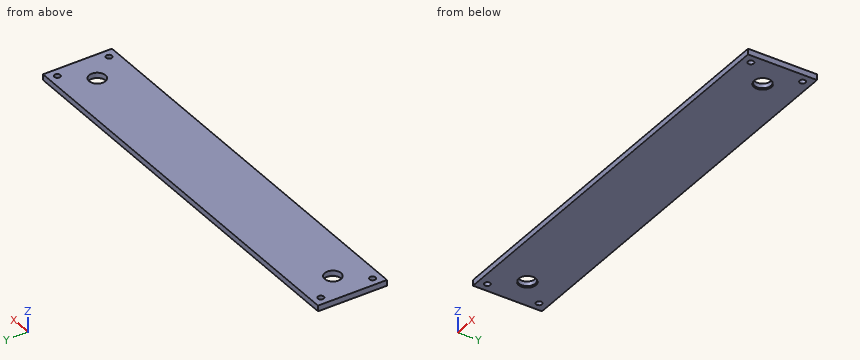
from build123d import *

# Parameters (mm, degrees)
SKETCH1_W           = 360
SKETCH1_H           = 60
SKETCH1_R           = 7.1
BOSS_EXTRUDE1_DEPTH = 4
SKETCH2_W           = 360
SKETCH2_H           = 60
SKETCH2_R           = 7.6
BOSS_EXTRUDE2_DEPTH = 1
CUT_EXTRUDE1_REACH  = 337.423
SKETCH3_R           = 2.55


with BuildPart() as part:
    # Sketch1 → Boss-Extrude1 (new body)
    with BuildSketch(Plane.XY):
        with Locations((-154.041275094, 0)):
            Rectangle(SKETCH1_W, SKETCH1_H)
        Circle(SKETCH1_R, mode=Mode.SUBTRACT)
        with Locations((-308.082550187, -0.2)):
            Circle(SKETCH1_R, mode=Mode.SUBTRACT)
    extrude(amount=-BOSS_EXTRUDE1_DEPTH)

    # Sketch2 → Boss-Extrude2 (add)
    with BuildSketch(Plane(origin=(0, 0, -4), x_dir=(-1, 0, 0), z_dir=(0, 0, -1))):
        with Locations((154.041275094, 0)):
            Rectangle(SKETCH2_W, SKETCH2_H)
        Circle(SKETCH2_R, mode=Mode.SUBTRACT)
        with Locations(Location((308.082550187, 0, 0), (0, 0, 180))):
            Circle(SKETCH2_R, mode=Mode.SUBTRACT)
    extrude(amount=BOSS_EXTRUDE2_DEPTH)

    # Sketch3 → Cut-Extrude1 (cut, up to next)
    with BuildSketch(Plane(origin=(0, 0, -5), x_dir=(-1, 0, 0), z_dir=(0, 0, -1)), mode=Mode.PRIVATE) as cut_extrude1_sk1:
        with Locations((326.53392807, -22.492652976)):
            Circle(SKETCH3_R)
    cut_extrude1_tool1 = extrude(cut_extrude1_sk1.sketch, amount=-CUT_EXTRUDE1_REACH, mode=Mode.PRIVATE) & part.part
    # Sketch3 → Cut-Extrude1 (cut, up to next)
    with BuildSketch(Plane(origin=(0, 0, -5), x_dir=(-1, 0, 0), z_dir=(0, 0, -1)), mode=Mode.PRIVATE) as cut_extrude1_sk2:
        with Locations((326.53392807, 22.492652976)):
            Circle(SKETCH3_R)
    cut_extrude1_tool2 = extrude(cut_extrude1_sk2.sketch, amount=-CUT_EXTRUDE1_REACH, mode=Mode.PRIVATE) & part.part
    # Sketch3 → Cut-Extrude1 (cut, up to next)
    with BuildSketch(Plane(origin=(0, 0, -5), x_dir=(-1, 0, 0), z_dir=(0, 0, -1)), mode=Mode.PRIVATE) as cut_extrude1_sk3:
        with Locations(Location((-18.451377883, -22.492652976, 0), (0, 0, 180))):
            Circle(SKETCH3_R)
    cut_extrude1_tool3 = extrude(cut_extrude1_sk3.sketch, amount=-CUT_EXTRUDE1_REACH, mode=Mode.PRIVATE) & part.part
    # Sketch3 → Cut-Extrude1 (cut, up to next)
    with BuildSketch(Plane(origin=(0, 0, -5), x_dir=(-1, 0, 0), z_dir=(0, 0, -1)), mode=Mode.PRIVATE) as cut_extrude1_sk4:
        with Locations((-18.451377883, 22.492652976)):
            Circle(SKETCH3_R)
    cut_extrude1_tool4 = extrude(cut_extrude1_sk4.sketch, amount=-CUT_EXTRUDE1_REACH, mode=Mode.PRIVATE) & part.part
    add(cut_extrude1_tool1.solids().sort_by_distance((-326.533928, -22.492653, -5))[0], mode=Mode.SUBTRACT)
    add(cut_extrude1_tool2.solids().sort_by_distance((-326.533928, 22.492653, -5))[0], mode=Mode.SUBTRACT)
    add(cut_extrude1_tool3.solids().sort_by_distance((18.451378, -22.492653, -5))[0], mode=Mode.SUBTRACT)
    add(cut_extrude1_tool4.solids().sort_by_distance((18.451378, 22.492653, -5))[0], mode=Mode.SUBTRACT)


solid = part.part
Work out the finished part from the listing and answer in its coordinate system (mm). Round coordinates to 2 decimals unless told otherwise and drop trailing zeros. Write each loop counter-clockwise with the first axis right and the second up, starting at its lowest first coordinate (ties: lowest second). Pieces come first, ordered by that corner, then holes. Notation, with made-up numbers: (56, 80.25) - (101, 80.25) arc R24 ccw to (101, 110.25) - close; hole circle Ø3 at (47, 86.5). An arc over 180 degrees is marked (long way). Answer in a Markdown table with one row per item. Add a question column.
1. A cutting plane is placed at B-B, the plane z = -2.75. Determine the outline of the cut face in (x, y).
2. A cutting plane is placed at A-A, the plane x = 0. Determine the outline of the cut face in (y, z).
3. Find the intervals of material crossed by line 1 along X through (y, z) = (0.5, -3); line 2 along X through (y, z) = (-1, -1.85); line 3 along Y through (x, z) = (0, -4.45), in increasing order. Write a range as from..to.
Worked out:
| question | item | result |
|---|---|---|
| 1 | outline | (-334.04, -30) - (25.96, -30) - (25.96, 30) - (-334.04, 30) - close; hole circle Ø5.1 at (-326.53, -22.49); hole circle Ø5.1 at (-326.53, 22.49); hole circle Ø14.2 at (-308.08, -0.2); hole circle Ø14.2 at (0, 0); hole circle Ø5.1 at (18.45, -22.49); hole circle Ø5.1 at (18.45, 22.49) |
| 2 | outline | (-30, -5) - (-7.6, -5) - (-7.6, -4) - (-7.1, -4) - (-7.1, 0) - (-30, 0) - close; (7.1, -4) - (7.6, -4) - (7.6, -5) - (30, -5) - (30, 0) - (7.1, 0) - close |
| 3 | line 1 | -334.04..-315.15, -301.02..-7.08, 7.08..25.96 |
| 3 | line 2 | -334.04..-315.14, -301.03..-7.03, 7.03..25.96 |
| 3 | line 3 | -30..-7.6, 7.6..30 |
